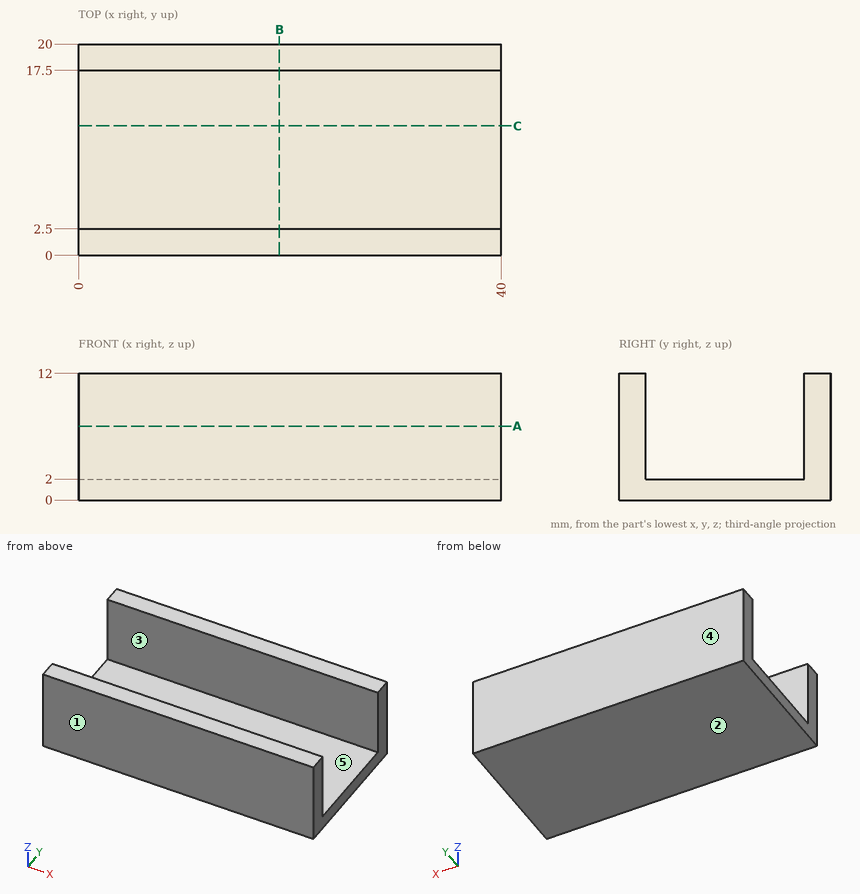
The drawing under review shows one solid part. Ordinate dimensions are in mm from its lowest x, y, z. A direction names the side the tool comes from. Round coordinates to 2 decimals unless told otherwise and drop trailing zeros. Order: outer loops, then holes, each group sorted by start corner. A loop starts at its lowest first (then second) coordinate and runs counter-clockwise, first axis right, second up. Notation, with made-up numbers: (24.5, 75.25) -> (40.5, 75.25) arc R33 cw to (40.5, 104.25) -> close; hole circle Ø4 at (-3, 36.5). An arc over 180 degrees is marked (long way). Use a Markdown table: item, result.
Q1. We need section A-A on z = 7. Write out the cut boundary in (x, y), then the cut area to 3 significant figures.
Values:
| item | result |
|---|---|
| outline | (0, 0) -> (40, 0) -> (40, 2.5) -> (0, 2.5) -> close; (0, 17.5) -> (40, 17.5) -> (40, 20) -> (0, 20) -> close |
| area | 200 mm^2 |
Q2. For line 1 (Y direction, x = 30, z = 4.25); line 2 (Z direction, x = 24, y = 5.25), list the stretches that pass through material, from the lowest coordinate up.
Values:
| item | result |
|---|---|
| line 1 | y = 0 to 2.5, 17.5 to 20 |
| line 2 | z = 0 to 2 |
Q3. We need section C-C on y = 12.25. Write out the cut boundary in (x, z), then the cut area to 3 significant figures.
Values:
| item | result |
|---|---|
| outline | (0, 0) -> (40, 0) -> (40, 2) -> (0, 2) -> close |
| area | 80.0 mm^2 |
Q4. Tool access review of the marked faces 4 and 5: name each direction out of +Z, -Z, +X, -X, +Y, -Y from which nothing blocks a thin tool from reaching the whole face with its end or side.
Values:
| item | result |
|---|---|
| face 4 | +Z, -Z, +X, -X, +Y |
| face 5 | +Z, +X, -X |
Q5. Mouldability with a two-part tool opening along Y and no side actions: class the marked faces 1, 2 and 3 as +Y half, -Y half, draft (parallel to the pull), parting line (faces both ways), or undercut.
Values:
| item | result |
|---|---|
| face 1 | -Y half |
| face 2 | draft |
| face 3 | undercut |
Q6. Clearance check with a flat-ended pin moving along its axis: P1, Ø2, axis at x = 19.5, y = 11, coming from the +Z side. State where the tip first meets the part, or that it passes through.
Values:
| item | result |
|---|---|
| P1 | stops at z = 2 |
Q7. We need section B-B on x = 19. Write out the cut boundary in (y, z), then the cut area to 3 significant figures.
Values:
| item | result |
|---|---|
| outline | (0, 0) -> (20, 0) -> (20, 12) -> (17.5, 12) -> (17.5, 2) -> (2.5, 2) -> (2.5, 12) -> (0, 12) -> close |
| area | 90.0 mm^2 |
